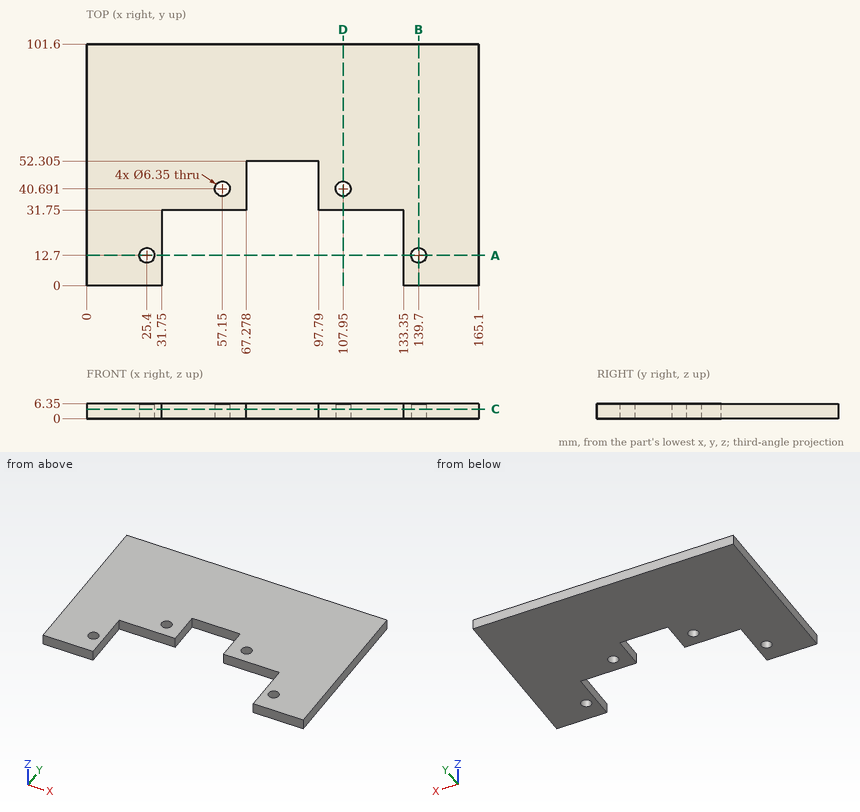
Source: three-view drawing plus pictorial views. Frame: mm from the lowest corner of the part. Coordinates: 2 decimals unless noted, no trailing zeros. Write each loop counter-clockwise with the first axis right and the second up, starting at its lowest first coordinate (ties: lowest second). Pieces come first, ordered by that corner, then holes. Notation, with made-up numbers: (-31.5, 65.5) -> (-6.5, 65.5) arc R20 cw to (-6.5, 71.5) -> close; hole circle Ø11 at (20, 57). An arc over 180 degrees is marked (long way). Answer as a JSON object with one key per item and string values.
1. Section A-A on y = 12.7. Return the cut outline in (x, z) (3 decimals), then the cut area to 3 significant figures.
Result set:
{"outline": "(0, 0) -> (22.225, 0) -> (22.225, 6.35) -> (0, 6.35) -> close; (28.575, 0) -> (31.75, 0) -> (31.75, 6.35) -> (28.575, 6.35) -> close; (133.35, 0) -> (136.525, 0) -> (136.525, 6.35) -> (133.35, 6.35) -> close; (142.875, 0) -> (165.1, 0) -> (165.1, 6.35) -> (142.875, 6.35) -> close", "area": "323 mm2"}
2. First-contact query: P1, Ø1.9, axis at x = 116.5, z = 3, coming from the -Y side. Flat tip, straight axial feed; report the tip coordinate or a pass-through.
Result set:
{"P1": "stops at y = 31.75"}
3. Section C-C on z = 4. Count the separate pieces of the cut face and the enclosed holes in it, then the cut area to 3 significant figures.
Result set:
{"separate pieces": "1", "enclosed holes": "4", "area": "12,800 mm2"}
4. Material intervals for line 1 (X direction, y = 12.7, z = 3) (3 decimals); line 2 (X direction, y = 6, z = 5); line 3 (Y direction, x = 57.15, z = 3.25), sorted ascending. Write a range as from..to.
Result set:
{"line 1": "x = 0..22.225, 28.575..31.75, 133.35..136.525, 142.875..165.1", "line 2": "x = 0..31.75, 133.35..165.1", "line 3": "y = 31.75..37.52, 43.87..101.6"}
5. Section B-B on x = 139.7. Return the cut outline in (y, z) (3 decimals).
Result set:
{"outline": "(0, 0) -> (9.525, 0) -> (9.525, 6.35) -> (0, 6.35) -> close; (15.875, 0) -> (101.6, 0) -> (101.6, 6.35) -> (15.875, 6.35) -> close"}
6. Section D-D on x = 107.95. Return the cut outline in (y, z).
Result set:
{"outline": "(31.75, 0) -> (37.52, 0) -> (37.52, 6.35) -> (31.75, 6.35) -> close; (43.87, 0) -> (101.6, 0) -> (101.6, 6.35) -> (43.87, 6.35) -> close"}
